```python
from build123d import *

# Parameters (mm, degrees)
F1_DEPTH = 152.4
F2_W     = 113.335262984
F2_H     = 152.4
F3_DEPTH = 25.4


# Not quite as in the source:
# - a feature names something its author has since deleted; it is built from what else it names


with BuildPart() as f1:
    # F0 (on Front) → F1 (new body)
    with BuildSketch(Plane.XZ):
        Polygon((-61.8058890104, -21.7274855822), (-66.5037259459, -21.7274855822), (-66.5037259459, -32.5912311673), (-38.6103317142, -32.5912311673), (-38.6103317142, -21.7274855822), (-47.4187731743, -21.7274855822), (-47.4187731743, 39.9315953255), (38.9039441943, 39.9315953255), (38.9039441943, -21.7274855822), (25.6912820041, -21.7274855822), (25.6912820041, -32.5912311673), (59.7505830228, -32.5912311673), (59.7505830228, -21.7274855822), (51.5293739736, -21.7274855822), (51.5293739736, 50.5017265677), (-61.8058890104, 50.5017265677), align=None)
    extrude(amount=F1_DEPTH)

    # F2 (on face) → F3 (join)
    with BuildSketch(Plane.XY.offset(50.5017265677)):
        with Locations((-5.1382575184, -76.2)):
            Rectangle(F2_W, F2_H)
        with BuildLine():
            Line((-31.2988758087, -123.7941682339), (-31.2988758087, -34.4304777682))
            ThreePointArc((-31.2988758087, -34.4304777682), (-5.1382575184, -8.2698594779), (21.0223607719, -34.4304777682))
            Line((21.0223607719, -34.4304777682), (21.0223607719, -123.7941682339))
            ThreePointArc((21.0223607719, -123.7941682339), (-5.1382575184, -149.9547865242), (-31.2988758087, -123.7941682339))
        make_face(mode=Mode.SUBTRACT)
    extrude(amount=F3_DEPTH)


solid = f1.part
```
Check sheet for the modelled part. Datum: model origin and axes. Units: mm. A direction names the side the tool comes from. Give positions to 0.01 mm unless a question says otherwise; leave off trailing zeros. Write each loop counter-clockwise with the first axis right and the second up, starting at its lowest first coordinate (ties: lowest second). Pieces come first, ordered by that corner, then holes.
Item 1: Scan lines: L1, parallel to X at y = -69.5, z = -22; L2, parallel to X at y = -25.5, z = 31.5; L3, parallel to Z at x = 34.5, y = -33.5. Record each from-to range of solid material in increasing order.
Item 2: Cross-section at C-C (z = 56). Enter the section's corners in (x, y).
Item 3: Draft check along Z on faces 1 (the face through (-47.419, -75, 9)), 2 (the face through (-5, -78, 50.502)), 3 (the face through (-5.714, -8.276, 63.024)). Enter one of: released by +Z, released by -Z, zero draft, split by the parting line, or undercut.
Item 4: Gauge pin test, flat ends, axial feed: pin 1 (7.5 mm diameter, centred on y = -91, z = 63, fed in from -X); pin 2 (10 mm diameter, centred on x = -9.5, y = -58, fed in from -Z); pin 3 (1.4 mm diameter, centred on x = -63.5, y = -48.5, fed in from +Z). Record the tip position at first contact, or that the pin passes through.
Item 5: Access from +Z, -Z, +X, -X, +Y, -Y to the whole of each face (thin tool, end or side, straight path). Record for faces 4 (the face through (-4.56, -149.95, 63.02)), 5 (the face through (56, -75, -21.727)), 6 (the face through (-61.806, -77, 26)), 7 (the face through (32, -75, -21.727)).
Item 6: Cross-section at A-A (z = 33). Enter the section's corners in (x, y), and give its area (3 significant figures).
Item 7: Cross-section at B-B (x = 36). Enter the section's corners in (y, z).
Item 8: Cross-section at D-D (y = -42.5). Enter the section's corners in (x, z).
Report:
1. L1: x = -66.5 to -38.61, 25.69 to 59.75
1. L2: x = -61.81 to -47.42, 38.9 to 51.53
1. L3: z = -32.59 to -21.73, 39.93 to 75.9
2. outline: (-61.81, -152.4) - (51.53, -152.4) - (51.53, 0) - (-61.81, 0) - close; hole (-31.3, -123.79) arc R26.16 ccw to (21.02, -123.79) - (21.02, -34.43) arc R26.16 ccw to (-31.3, -34.43) - close
3. face 1: undercut
3. face 2: released by +Z
3. face 3: zero draft
4. pin 1: stops at x = -61.81
4. pin 2: stops at z = 39.93
4. pin 3: stops at z = -21.73
5. face 4: +Z
5. face 5: +Z, +X, +Y, -Y
5. face 6: +Z, -X, +Y, -Y
5. face 7: +Y, -Y
6. outline: (-61.81, -152.4) - (-47.42, -152.4) - (-47.42, 0) - (-61.81, 0) - close; (38.9, -152.4) - (51.53, -152.4) - (51.53, 0) - (38.9, 0) - close
6. area: 4,120 mm2
7. outline: (-152.4, -32.59) - (0, -32.59) - (0, -21.73) - (-152.4, -21.73) - close; (-152.4, 39.93) - (0, 39.93) - (0, 75.9) - (-152.4, 75.9) - close
8. outline: (-66.5, -32.59) - (-38.61, -32.59) - (-38.61, -21.73) - (-47.42, -21.73) - (-47.42, 39.93) - (38.9, 39.93) - (38.9, -21.73) - (25.69, -21.73) - (25.69, -32.59) - (59.75, -32.59) - (59.75, -21.73) - (51.53, -21.73) - (51.53, 75.9) - (21.02, 75.9) - (21.02, 50.5) - (-31.3, 50.5) - (-31.3, 75.9) - (-61.81, 75.9) - (-61.81, -21.73) - (-66.5, -21.73) - close
